Source: CAD feature listing. Evaluate the final solid. Frame: model axes, mm. A direction names the side the tool comes from. Give positions to 0.01 mm unless a question says otherwise; leave off trailing zeros. Write each loop counter-clockwise with the first axis right and the second up, starting at its lowest first coordinate (ties: lowest second). Pieces come first, ordered by that corner, then holes. Notation, with made-up numbers: (-36, 57) - (-1, 57) arc R20 ccw to (-1, 93) - close; hole circle Ø10 at (-4, 69). An arc over 180 degrees is marked (long way). One line per question, with ' | ' between items. Start each with the question number.
(1) Section A-A, the plane y = -2.65. Return loops of the section in (x, z), plus the area to 3 significant figures.
(2) Section D-D, the plane z = 6.25. Return loops of the section in (x, y).
(3) Section B-B, the plane z = 0. Return loops of the section in (x, y), plus the area to 4 significant figures.
(4) Draft query along X for faces 1 (the cylindrical face through (-7.62, -0.74, -3.16)), 2 (the flat face through (-3.45, -3.27, 6.09)), 3 (the flat face through (4, -1.5, -6)), 4 (the cylindrical face through (6, -2, 0)). Return one class per face: +X half, -X half, draft (parallel to the pull), parting line (faces both ways), or undercut.
(5) Access query for faces 5 (the flat face through (3.45, -3.27, -6.09)), 6 (the flat face through (3.549, -3.274, 6.034)), 7 (the flat face through (-7, -3, 0)), 8 (the flat face through (7, -3, 0)), 9 (the flat face through (-3.549, -3.274, -6.034)). Directions: +Z, -Z, +X, -X, +Y, -Y. A direction counts if a zero-diameter tool reaches every point of the face in a straight line with its end or side. Return the directions, or none.
(6) Ray query, line 1 (Z direction, x = 0, y = -0.95); line 2 (X direction, y = -3.05, z = 3.75); line 3 (X direction, y = -1, z = -3.25). Return the intervals inside material, ascending. Write a range as [from, to].
(7) Pin query (flat end, axial travel): pin 1 (4 mm diameter, centred on x = -6, z = 6.5, fed in from +Y); pin 2 (3 mm diameter, centred on y = -4, z = 1, fed in from -X); pin 3 (1 mm diameter, centred on y = -1.5, z = -6.5, fed in from +X); pin 4 (2 mm diameter, centred on x = -3.5, y = -0.5, fed in from +Z). Return the tip coordinate at first contact, or that it passes through.
(8) Section C-C, the plane x = 4. Return loops of the section in (y, z), plus the area to 3 significant figures.
```python
from build123d import *

# Parameters (mm, degrees)
SKETCH1_W          = 2.25
SKETCH1_H          = 5
SKETCH2_R          = 8.25
CUT_EXTRUDE1_DEPTH = 3.5


with BuildPart() as part:
    # Sketch1 → Revolve1 (revolve)
    with BuildSketch(Plane.XY):
        with Locations((-7.125, -2.5)):
            Rectangle(SKETCH1_W, SKETCH1_H)
    revolve(axis=Axis((0, -3.49659483, 0), (0, 1, 0)))

    # Sketch2 → Cut-Extrude1 (cut)
    with BuildSketch(Plane.XZ.offset(5)):
        Circle(SKETCH2_R)
        Polygon((0, 8.082903769), (-7, 4.041451884), (-7, -4.041451884), (0, -8.082903769), (7, -4.041451884), (7, 4.041451884), align=None, mode=Mode.SUBTRACT)
    extrude(amount=-CUT_EXTRUDE1_DEPTH, mode=Mode.SUBTRACT)


solid = part.part
```
Check sheet entries:
1) outline: (-7, -4.04) - (0, -8.08) - (7, -4.04) - (7, 4.04) - (0, 8.08) - (-7, 4.04) - close; hole circle Ø12 at (0, 0) | area: 56.6 mm²
2) outline: (-5.39, -1.5) - (-3.17, -1.5) - (-3.17, -5) - (3.17, -5) - (3.17, -1.5) - (5.39, -1.5) - (5.39, 0) - (-5.39, 0) - close
3) outline: (-8.25, -1.5) - (-7, -1.5) - (-7, -5) - (-6, -5) - (-6, 0) - (-8.25, 0) - close; (6, -5) - (7, -5) - (7, -1.5) - (8.25, -1.5) - (8.25, 0) - (6, 0) - close | area: 13.75 mm²
4) face 1: parting line | face 2: -X half | face 3: draft | face 4: undercut
5) face 5: -Z, +X, -Y | face 6: +Z, +X, -Y | face 7: +Z, -Z, -X, -Y | face 8: +Z, -Z, +X, -Y | face 9: -Z, -X, -Y
6) line 1: [-8.25, -6], [6, 8.25] | line 2: [-7, -4.68], [4.68, 7] | line 3: [-7.58, -5.04], [5.04, 7.58]
7) pin 1: y = 0 | pin 2: x = -7 | pin 3: x = 5.66 | pin 4: z = 7.86
8) outline: (-5, -5.77) - (-1.5, -5.77) - (-1.5, -7.22) - (0, -7.22) - (0, -4.47) - (-5, -4.47) - close; (-5, 4.47) - (0, 4.47) - (0, 7.22) - (-1.5, 7.22) - (-1.5, 5.77) - (-5, 5.77) - close | area: 17.3 mm²
